Work out the finished part from the listing and answer in its coordinate system (mm). Face numbers are marked on the shaded views. Round coordinates to 2 decimals unless told otherwise and drop trailing zeros. Loops run counter-clockwise (first coordinate to the right, second up) from the corner with the lowest first, then second, coordinate; pieces in that order, holes last.
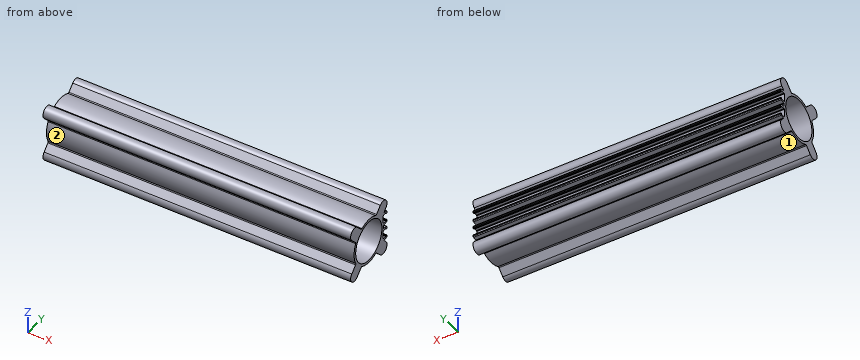
Autodesk Inventor part; units mm, degrees
ref_plane "br_l_XY" through (0, 0, 0) normal (1, 0, 0) x (0, 0, -1)
ref_plane "br_l_YZ" through (0, 0, 0) normal (0, 0, -1) x (0, 1, 0)
ref_plane "br_l_ZX" through (0, 0, 0) normal (0, 1, 0) x (1, 0, 0)
sketch "Sketch_1" plane through (0, 0, 0) normal (1, 0, 0) x (0, 1, 0)
  arc A0 (-14.0912, 20.8088) -> (-20.8088, 14.0912) centre (-17.45, 17.45) ccw
  line L0 (-20.8088, 14.0912) -> (-16.1638, 9.4463)
  arc A1 (-15.9829, 8.2792) -> (-16.1638, 9.4463) centre (-16.8709, 8.7392) ccw
  arc A2 (-15.9829, 8.2792) -> (-15.983, -8.2792) centre (0, 0) ccw
  arc A3 (-16.1638, -9.4463) -> (-15.983, -8.2792) centre (-16.8709, -8.7392) ccw
  line L1 (-16.1638, -9.4463) -> (-20.8088, -14.0912)
  arc A4 (-20.8088, -14.0912) -> (-14.0912, -20.8088) centre (-17.45, -17.45) ccw
  line L2 (-14.0912, -20.8088) -> (-9.4463, -16.1638)
  arc A5 (-8.2792, -15.9829) -> (-9.4463, -16.1638) centre (-8.7392, -16.8709) ccw
  arc A6 (-8.2792, -15.9829) -> (8.2792, -15.983) centre (0, 0) ccw
  arc A7 (9.4463, -16.1638) -> (8.2792, -15.983) centre (8.7392, -16.8709) ccw
  line L3 (9.4463, -16.1638) -> (14.0912, -20.8088)
  arc A8 (14.0912, -20.8088) -> (20.8088, -14.0912) centre (17.45, -17.45) ccw
  line L4 (20.8088, -14.0912) -> (18.7215, -12.004)
  arc A9 (18.8549, -11.581) -> (18.7215, -12.004) centre (18.8983, -11.8272) ccw
  line L5 (18.8549, -11.581) -> (21.6129, -11.0947)
  arc A10 (21.6129, -11.0947) -> (22.15, -10.4546) centre (21.5, -10.4546) ccw
  line L6 (22.15, -10.4546) -> (22.15, -9.625)
  arc A11 (22.15, -9.625) -> (21.75, -9.225) centre (21.75, -9.625) ccw
  line L7 (21.75, -9.225) -> (20.9499, -9.225)
  line L8 (20.9499, -9.225) -> (20.9499, -9.9)
  line L9 (20.9499, -9.9) -> (17.9999, -9.9)
  arc A12 (17.5999, -9.5) -> (17.9999, -9.9) centre (17.9999, -9.5) ccw
  line L10 (17.5999, -9.5) -> (17.5999, -3.5)
  arc A13 (17.9999, -3.1) -> (17.5999, -3.5) centre (17.9999, -3.5) ccw
  line L11 (17.9999, -3.1) -> (20.9499, -3.1)
  line L12 (20.9499, -3.1) -> (20.9499, -3.775)
  line L13 (20.9499, -3.775) -> (21.75, -3.775)
  arc A14 (21.75, -3.775) -> (22.15, -3.375) centre (21.75, -3.375) ccw
  line L14 (22.15, -3.375) -> (22.15, -2.5454)
  arc A15 (22.15, -2.5454) -> (21.6129, -1.9053) centre (21.5, -2.5454) ccw
  line L15 (21.6129, -1.9053) -> (18.3939, -1.3377)
  arc A16 (17.9812, -0.8224) -> (18.3939, -1.3377) centre (18.4807, -0.8453) ccw
  arc A17 (17.9812, -0.8224) -> (17.9812, 0.8224) centre (0, 0) ccw
  arc A18 (18.3939, 1.3377) -> (17.9812, 0.8224) centre (18.4807, 0.8453) ccw
  line L16 (18.3939, 1.3377) -> (21.6129, 1.9053)
  arc A19 (21.6129, 1.9053) -> (22.15, 2.5454) centre (21.5, 2.5454) ccw
  line L17 (22.15, 2.5454) -> (22.15, 3.375)
  arc A20 (22.15, 3.375) -> (21.75, 3.775) centre (21.75, 3.375) ccw
  line L18 (21.75, 3.775) -> (20.9499, 3.775)
  line L19 (20.9499, 3.775) -> (20.9499, 3.1)
  line L20 (20.9499, 3.1) -> (17.9999, 3.1)
  arc A21 (17.5999, 3.5) -> (17.9999, 3.1) centre (17.9999, 3.5) ccw
  line L21 (17.5999, 3.5) -> (17.5999, 9.5)
  arc A22 (17.9999, 9.9) -> (17.5999, 9.5) centre (17.9999, 9.5) ccw
  line L22 (17.9999, 9.9) -> (20.9499, 9.9)
  line L23 (20.9499, 9.9) -> (20.9499, 9.225)
  line L24 (20.9499, 9.225) -> (21.75, 9.225)
  arc A23 (21.75, 9.225) -> (22.15, 9.625) centre (21.75, 9.625) ccw
  line L25 (22.15, 9.625) -> (22.15, 10.4546)
  arc A24 (22.15, 10.4546) -> (21.6129, 11.0947) centre (21.5, 10.4546) ccw
  line L26 (21.6129, 11.0947) -> (18.8549, 11.581)
  arc A25 (18.7215, 12.004) -> (18.8549, 11.581) centre (18.8983, 11.8272) ccw
  line L27 (18.7215, 12.004) -> (20.8088, 14.0912)
  arc A26 (20.8088, 14.0912) -> (14.0912, 20.8088) centre (17.45, 17.45) ccw
  line L28 (14.0912, 20.8088) -> (9.4463, 16.1638)
  arc A27 (8.2792, 15.983) -> (9.4463, 16.1638) centre (8.7392, 16.8709) ccw
  arc A28 (8.2792, 15.983) -> (-8.2792, 15.983) centre (0, 0) ccw
  arc A29 (-9.4463, 16.1638) -> (-8.2792, 15.983) centre (-8.7392, 16.8709) ccw
  line L29 (-9.4463, 16.1638) -> (-14.0912, 20.8088)
  circle A30 centre (0, 0) radius 16
extrude "Extrusion1" add sketch "Sketch_1" along normal blind 242
ref_plane "br_l_XY" through (0, 0, 0) normal (1, 0, 0) x (0, 0, -1)
ref_plane "br_l_YZ" through (0, 0, 0) normal (0, 0, -1) x (0, 1, 0)
ref_plane "br_l_ZX" through (0, 0, 0) normal (0, 1, 0) x (1, 0, 0)
ref_plane "br_r_XY" through (242, 0, 0) normal (-1, 0, 0) x (0, 0, -1)
ref_plane "br_r_YZ" through (242, 0, 0) normal (0, 0, -1) x (0, -1, 0)
ref_plane "br_r_ZX" through (242, 0, 0) normal (0, -1, 0) x (-1, 0, 0)
ref_plane "mod_en_XY" through (121, 0, 0) normal (1, 0, 0) x (0, 0, -1)
ref_plane "mod_en_YZ" through (121, 0, 0) normal (0, 0, -1) x (0, 1, 0)
ref_plane "mod_en_ZX" through (121, 0, 0) normal (0, 1, 0) x (1, 0, 0)
ref_plane "sens_sqr_l_XY" through (0, 17.6, -6.5) normal (-1, 0, 0) x (0, 0, -1)
ref_plane "sens_sqr_l_YZ" through (0, 17.6, -6.5) normal (0, 0, -1) x (0, -1, 0)
ref_plane "sens_sqr_l_ZX" through (0, 17.6, -6.5) normal (0, -1, 0) x (-1, 0, 0)
ref_plane "sens_sqr_r_XY" through (242, 17.6, 6.5) normal (1, 0, 0) x (0, 0, -1)
ref_plane "sens_sqr_r_YZ" through (242, 17.6, 6.5) normal (0, 0, -1) x (0, 1, 0)
ref_plane "sens_sqr_r_ZX" through (242, 17.6, 6.5) normal (0, 1, 0) x (1, 0, 0)
ref_plane "sensor_l_XY" through (2.7, 19.65, -6.5) normal (0, -1, 0) x (1, 0, 0)
ref_plane "sensor_l_YZ" through (2.7, 19.65, -6.5) normal (1, 0, 0) x (0, 0, 1)
ref_plane "sensor_l_ZX" through (2.7, 19.65, -6.5) normal (0, 0, 1) x (0, -1, 0)
ref_plane "sensor_r_XY" through (239.3, 19.65, 6.5) normal (0, -1, 0) x (1, 0, 0)
ref_plane "sensor_r_YZ" through (239.3, 19.65, 6.5) normal (1, 0, 0) x (0, 0, 1)
ref_plane "sensor_r_ZX" through (239.3, 19.65, 6.5) normal (0, 0, 1) x (0, -1, 0)
properties part number "32-121-200--173-s3"
1. Consider probe 1 along Z at (x, y) = (125.5, 0); probe 2 along Y at (x, z) = (22.5, -9.5); probe 3 along Y at (x, z) = (172, -3.5). Determine where each line is inside the solid, lowest interval first.
Answer key:
probe 1: z = -18 to -16, 16 to 18
probe 2: y = -16.22 to -12.87, 12.87 to 17.6, 20.95 to 22.13
probe 3: y = -17.66 to -15.61, 15.61 to 17.6, 20.95 to 22.13
2. Find section B-B (z = 6). Write down the section's boundary in (x, y).
Answer key:
outline: (0, -16.97) - (242, -16.97) - (242, -14.83) - (0, -14.83) - close; (0, 14.83) - (242, 14.83) - (242, 17.6) - (0, 17.6) - close
3. Find section A-A (y = 0). Write down the section's boundary in (x, z), then the cut area to 3 significant figures.
Answer key:
outline: (0, -18) - (242, -18) - (242, -16) - (0, -16) - close; (0, 16) - (242, 16) - (242, 18) - (0, 18) - close
area: 968 mm2
4. Determine the mould class of the marked faces 1 and 2 for opening direction Y: +Y half, -Y half, draft (parallel to the pull), parting line (faces both ways), or undercut.
Answer key:
face 1: undercut
face 2: -Y half
5. Given pin 1 (2.5 mm diameter, centred on x = 113, y = 19.5, fed in from -Z); pin 2 (0.9 mm diameter, centred on x = 79, y = 21.5, fed in from +Z); pin 3 (5 mm diameter, centred on x = 85.5, y = -11, fed in from -Z); pin 4 (2 mm diameter, centred on y = -8.5, z = -11, fed in from +X), each flat-ended and moving along its own axis, determine where each tip first touches the part or whether it passes through.
Answer key:
pin 1: stops at z = -22.13
pin 2: stops at z = 20.55
pin 3: stops at z = -20.22
pin 4: passes through
